Read the model definition and answer for the solid it produces. Units are mm, in the model's axes. Give positions to 0.01 mm unless a question says otherwise; leave off trailing zeros. Write each loop counter-clockwise with the first axis right and the second up, starting at its lowest first coordinate (ties: lowest second). Pieces come first, ordered by that corner, then holes.
```python
from build123d import *

# Parameters (mm, degrees)
SKETCH1_R           = 1.85
BOSS_EXTRUDE1_DEPTH = 4.318


with BuildPart() as part:
    # Sketch1 → Boss-Extrude1 (new body)
    with BuildSketch(Plane.XY):
        with BuildLine():
            Line((47.48, 175), (47.48, 74.903475932))
            Line((47.48, 74.903475932), (-12.077446035, 74.903475932))
            Line((-12.077446035, 74.903475932), (-35.842451234, 116.06567238))
            Line((-35.842451234, 116.06567238), (-143, 127.288973426))
            Line((-143, 127.288973426), (-143, 211))
            Line((-143, 211), (143, 211))
            Line((143, 211), (143, 187))
            Line((143, 187), (59.48, 187))
            ThreePointArc((59.48, 187), (50.994718626, 183.485281374), (47.48, 175))
        make_face()
        with Locations((-134, 177.5)):
            Circle(SKETCH1_R, mode=Mode.SUBTRACT)
        with Locations((-126, 169.5)):
            Circle(SKETCH1_R, mode=Mode.SUBTRACT)
        with Locations((-126, 185.5)):
            Circle(SKETCH1_R, mode=Mode.SUBTRACT)
        with Locations((118, 200.5)):
            Circle(SKETCH1_R, mode=Mode.SUBTRACT)
        with Locations((126, 192.5)):
            Circle(SKETCH1_R, mode=Mode.SUBTRACT)
        with Locations((134, 200.5)):
            Circle(SKETCH1_R, mode=Mode.SUBTRACT)
    extrude(amount=BOSS_EXTRUDE1_DEPTH)


solid = part.part
```
Item 1: Section C-C (y = 136.5) is taken. Write down the section's boundary in (x, z), and give its area (3 significant figures).
Result set:
outline: (-143, 0) - (47.48, 0) - (47.48, 4.32) - (-143, 4.32) - close
area: 822 mm2
Item 2: Find the intervals of material crossed by line 1 along X through (y, z) = (200.5, 1.75); line 2 along X through (y, z) = (192.5, 2.7); line 3 along Y through (x, z) = (118, 1.2), in increasing order.
Result set:
line 1: x = -143 to 116.15, 119.85 to 132.15, 135.85 to 143
line 2: x = -143 to 124.15, 127.85 to 143
line 3: y = 187 to 198.65, 202.35 to 211
Item 3: Each of these flat-tipped pins is pushed along its axis until it touches: pin 1 Ø2 at (y, z) = (149, 2.5) entering from +X; pin 2 Ø2 at (y, z) = (107, 1.5) entering from -X. Where does it stop, or does it pass through?
Result set:
pin 1: stops at x = 47.48
pin 2: stops at x = -31.19
Item 4: Section B-B (x = 106) is taken. Write down the section's boundary in (y, z).
Result set:
outline: (187, 0) - (211, 0) - (211, 4.32) - (187, 4.32) - close
Item 5: Section A-A (z = 1.5) is taken. Write down the section's boundary in (x, y), and give its area (3 significant figures).
Result set:
outline: (-143, 127.29) - (-35.84, 116.07) - (-12.08, 74.9) - (47.48, 74.9) - (47.48, 175) arc R12 cw to (59.48, 187) - (143, 187) - (143, 211) - (-143, 211) - close; hole circle Ø3.7 at (-134, 177.5); hole circle Ø3.7 at (-126, 169.5); hole circle Ø3.7 at (-126, 185.5); hole circle Ø3.7 at (118, 200.5); hole circle Ø3.7 at (126, 192.5); hole circle Ø3.7 at (134, 200.5)
area: 22,700 mm2
